CAD build for the part. Positions are in the model's coordinates, mm. A direction names the side the tool comes from. Coordinates: 2 decimals unless noted, no trailing zeros. Write each loop counter-clockwise with the first axis right and the second up, starting at its lowest first coordinate (ties: lowest second). Pieces come first, ordered by that corner, then holes. Notation, with made-up numbers: M -8.5,-33 L 0.5,-33 A22 cw 0.5,-8 Z; hole C 21,41 d8. An arc over 180 degrees is marked long. Put each result on its own line as item: value. Start each with the question number.
```python
from build123d import *

# Parameters (mm, degrees)
F0_W     = 21
F0_H     = 37
F0_R     = 6
F0_H_2   = 4
F1_DEPTH = 5
F2_DEPTH = 45
F3_R     = 1.75
F4_DEPTH = 5
F5_R     = 1.3
F6_DEPTH = 10


with BuildPart() as f1:
    # F0 (on Top) → F1 (new body)
    with BuildSketch(Plane.XY):
        with Locations((3.617266193, -10.4946532761)):
            Rectangle(F0_W, F0_H)
        with Locations((3.617266193, -10.4946532761)):
            Circle(F0_R, mode=Mode.SUBTRACT)
        Polygon((16.117266193, 12.0053467239), (-8.882733807, 12.0053467239), (-8.882733807, 8.0053467239), (-6.882733807, 8.0053467239), (14.117266193, 8.0053467239), (16.117266193, 8.0053467239), align=None)
        Polygon((-6.882733807, 8.0053467239), (-8.882733807, 8.0053467239), (-8.882733807, -32.9946532761), (-6.882733807, -32.9946532761), (-6.882733807, -28.9946532761), align=None)
        Polygon((16.117266193, -32.9946532761), (16.117266193, 8.0053467239), (14.117266193, 8.0053467239), (14.117266193, -28.9946532761), (14.117266193, -32.9946532761), align=None)
        with Locations((3.617266193, -30.9946532761)):
            Rectangle(F0_W, F0_H_2)
    extrude(amount=F1_DEPTH)

    # F0 (on Top) → F2 (join)
    with BuildSketch(Plane.XY):
        Polygon((16.117266193, 12.0053467239), (-8.882733807, 12.0053467239), (-8.882733807, 8.0053467239), (-6.882733807, 8.0053467239), (14.117266193, 8.0053467239), (16.117266193, 8.0053467239), align=None)
        Polygon((-6.882733807, 8.0053467239), (-8.882733807, 8.0053467239), (-8.882733807, -32.9946532761), (-6.882733807, -32.9946532761), (-6.882733807, -28.9946532761), align=None)
        Polygon((16.117266193, -32.9946532761), (16.117266193, 8.0053467239), (14.117266193, 8.0053467239), (14.117266193, -28.9946532761), (14.117266193, -32.9946532761), align=None)
        with Locations((3.617266193, -30.9946532761)):
            Rectangle(F0_W, F0_H_2)
    extrude(amount=F2_DEPTH)

    # F3 (on face) → F4 (join)
    with BuildSketch(Plane(origin=(0, 12.0053467239, 0), x_dir=(-1, 0, 0), z_dir=(0, 1, 0))):
        with BuildLine():
            Line((-16.117266193, 35), (-16.117266193, 39))
            Line((-16.117266193, 39), (-20.117266193, 39))
            ThreePointArc((-20.117266193, 39), (-17.2888390683, 37.8284271247), (-16.117266193, 35))
        make_face()
        with BuildLine():
            Line((-16.117266193, 39), (-16.117266193, 45))
            Line((-16.117266193, 45), (-20.117266193, 45))
            Line((-20.117266193, 45), (-20.117266193, 43.75))
            ThreePointArc((-20.117266193, 43.75), (-18.879829326, 43.2374368671), (-18.367266193, 42))
            ThreePointArc((-18.367266193, 42), (-18.879829326, 40.7625631329), (-20.117266193, 40.25))
            Line((-20.117266193, 40.25), (-20.117266193, 39))
            Line((-20.117266193, 39), (-16.117266193, 39))
        make_face()
        with BuildLine():
            Line((-20.117266193, 43.75), (-20.117266193, 45))
            ThreePointArc((-20.117266193, 45), (-23.117266193, 42), (-20.117266193, 39))
            Line((-20.117266193, 39), (-20.117266193, 40.25))
            ThreePointArc((-20.117266193, 40.25), (-21.867266193, 42), (-20.117266193, 43.75))
        make_face()
        with BuildLine():
            Line((12.882733807, 45), (8.882733807, 45))
            Line((8.882733807, 45), (8.882733807, 39))
            Line((8.882733807, 39), (12.882733807, 39))
            ThreePointArc((12.882733807, 39), (15.882733807, 42), (12.882733807, 45))
        make_face()
        with Locations((12.882733807, 42)):
            Circle(F3_R, mode=Mode.SUBTRACT)
        with BuildLine():
            Line((12.882733807, 39), (8.882733807, 39))
            Line((8.882733807, 39), (8.882733807, 35))
            ThreePointArc((8.882733807, 35), (10.0543066822, 37.8284271247), (12.882733807, 39))
        make_face()
        with BuildLine():
            ThreePointArc((12.882733807, 0), (15.882733807, 3), (12.882733807, 6))
            Line((12.882733807, 6), (8.882733807, 6))
            Line((8.882733807, 6), (8.882733807, 0))
            Line((8.882733807, 0), (12.882733807, 0))
        make_face()
        with Locations((12.882733807, 3)):
            Circle(F3_R, mode=Mode.SUBTRACT)
        with BuildLine():
            ThreePointArc((12.882733807, 6), (10.0543066822, 7.1715728753), (8.882733807, 10))
            Line((8.882733807, 10), (8.882733807, 6))
            Line((8.882733807, 6), (12.882733807, 6))
        make_face()
        with BuildLine():
            Line((-16.117266193, 6), (-16.117266193, 10))
            ThreePointArc((-16.117266193, 10), (-17.2888390683, 7.1715728753), (-20.117266193, 6))
            Line((-20.117266193, 6), (-16.117266193, 6))
        make_face()
        with BuildLine():
            Line((-16.117266193, 6), (-20.117266193, 6))
            ThreePointArc((-20.117266193, 6), (-23.117266193, 3), (-20.117266193, 0))
            Line((-20.117266193, 0), (-16.117266193, 0))
            Line((-16.117266193, 0), (-16.117266193, 6))
        make_face()
        with Locations((-20.117266193, 3)):
            Circle(F3_R, mode=Mode.SUBTRACT)
    extrude(amount=-F4_DEPTH)

    # F5 (on face) → F6 (cut)
    with BuildSketch(Plane.XY.offset(45)):
        with Locations((3.617266193, 10.0053467239)):
            Circle(F5_R)
        with Locations((3.617266193, -30.9946532761)):
            Circle(F5_R)
    extrude(amount=-F6_DEPTH, mode=Mode.SUBTRACT)


solid = f1.part
```
(1) Drop flat-ended pins along their axis: pin 1 (4 mm diameter, centred on x = 20.12, z = 3, fed in from -Y); pin 2 (1.3 mm diameter, centred on x = 4, y = -31, fed in from +Z); pin 3 (11 mm diameter, centred on y = -16, z = 27.5, fed in from -X). Give the stop position or say it passes through.
(2) Slice it at A-A, the plane z = 14.5. Write the cut outline in (x, y), then the cut area to 3 significant figures.
(3) Slice it at D-D, the plane y = -5.5. Write the cut outline in (x, z).
(4) Which spindle directions (+Z, -Z, +X, -X, +Y, -Y) get a long thin tool onto all of the face, cutting with end or side? Do faces 1 (the face through (-10.023, 9.54, 37.797)), 2 (the face through (-10.8, 7.005, 2.8)), 3 (the face through (3.448, 11.294, 40.07)), 4 (the face through (17.32, 9.54, 37.86)). Say none if no direction does.
(5) Slice it at B-B, the plane z = 3. Write the cut outline in (x, y), then the cut area to 3 significant figures.
(6) Drill centre lines: line 1 (Y direction, x = 10.5, z = 7.5); line 2 (X direction, y = -14.5, z = 14); line 3 (X direction, y = 8.5, z = 41). Where is each one in solid material? Low to high. Write a range as [from, to].
(7) Slice it at C-C, the plane x = 7.5. Write the cut outline in (y, z).
(8) Two-plate mould, pull along Z, no slides. Class faces 5 (the face through (23.117, 9.54, 42.066)), 6 (the face through (18, 7.005, 42)), 7 (the face through (0, -5, 0)): +Z half, -Z half, draft (parallel to the pull), parting line (faces both ways), or undercut.
Result set:
1. pin 1: stops at y = 7.01
1. pin 2: stops at z = 35
1. pin 3: stops at x = -8.88
2. outline: M -8.88,-32.99 L 16.12,-32.99 L 16.12,12.01 L -8.88,12.01 Z; hole M -6.88,-28.99 L 14.12,-28.99 L 14.12,8.01 L -6.88,8.01 Z
2. area: 348 mm^2
3. outline: M -8.88,0 L 0.29,0 L 0.29,5 L -6.88,5 L -6.88,45 L -8.88,45 Z; M 6.94,0 L 16.12,0 L 16.12,45 L 14.12,45 L 14.12,5 L 6.94,5 Z
4. face 1: -X, +Y, -Y
4. face 2: +Z, -Z, -X, -Y
4. face 3: +Z
4. face 4: +X, +Y, -Y
5. outline: M -15.88,7.01 L -14.63,7.01 L -14.63,12.01 L -15.88,12.01 Z; M -11.13,7.01 L -8.88,7.01 L -8.88,-32.99 L 16.12,-32.99 L 16.12,7.01 L 18.37,7.01 L 18.37,12.01 L -11.13,12.01 Z; M 21.87,7.01 L 23.12,7.01 L 23.12,12.01 L 21.87,12.01 Z; hole C 3.62,-10.49 d12
5. area: 1,050 mm^2
6. line 1: y = [-32.99, -28.99], [8.01, 12.01]
6. line 2: x = [-8.88, -6.88], [14.12, 16.12]
6. line 3: x = [-15.71, -14.32], [-11.45, 18.68], [21.55, 22.95]
7. outline: M -32.99,0 L -15.07,0 L -15.07,5 L -28.99,5 L -28.99,45 L -32.99,45 Z; M -5.92,0 L 12.01,0 L 12.01,45 L 8.01,45 L 8.01,5 L -5.92,5 Z
8. face 5: undercut
8. face 6: draft
8. face 7: -Z half
